from build123d import *

# Parameters (mm, degrees)
BOSS_EXTRUDE1_DEPTH = 20
FILLET1_R           = 5
FILLET2_R           = 2
FILLET3_R           = 1.5
SKETCH4_R           = 2.9
CUT_EXTRUDE3_DEPTH  = 2
SKETCH5_R           = 1.625
CUT_EXTRUDE4_DEPTH  = 89.064050596
CUT_EXTRUDE5_DEPTH  = 2.3


with BuildPart() as part:
    # Sketch1 → Boss-Extrude1 (new body)
    with BuildSketch(Plane(origin=(0, 0, 0), x_dir=(1, 0, 0), z_dir=(0, 1, 0))):
        with BuildLine():
            Line((2.5, 62.713850172), (5.5, 62.713850172))
            Line((5.5, 62.713850172), (5.5, 52.713850172))
            ThreePointArc((5.5, 52.713850172), (0, -53), (-5.5, 52.713850172))
            Line((-5.5, 52.713850172), (-5.5, 62.713850172))
            Line((-5.5, 62.713850172), (-2.5, 62.713850172))
            Line((-2.5, 62.713850172), (-2.5, 49.937460889))
            ThreePointArc((-2.5, 49.937460889), (0, -50), (2.5, 49.937460889))
            Line((2.5, 49.937460889), (2.5, 62.713850172))
        make_face()
    extrude(amount=BOSS_EXTRUDE1_DEPTH)

    # Fillet1
    fillet1_edges = [part.edges().sort_by_distance(p)[0] for p in [
        (-2.5, 10, -49.937460889),
        (2.5, 10, -49.937460889),
    ]]
    fillet(fillet1_edges, radius=FILLET1_R)

    # Fillet2
    fillet2_edges = [part.edges().sort_by_distance(p)[0] for p in [
        (5.5, 10, -52.713850172),
        (-5.5, 10, -52.713850172),
    ]]
    fillet(fillet2_edges, radius=FILLET2_R)

    # Fillet3
    fillet3_edges = [part.edges().sort_by_distance(p)[0] for p in [
        (2.5, 0, -58.600043483),
        (0, 0, 50),
        (0, 20, 50),
        (-2.5, 0, -58.600043483),
        (-3.731108193, 0, -51.200593091),
        (3.731108193, 0, -51.200593091),
        (-2.5, 20, -58.600043483),
        (-3.731108193, 20, -51.200593091),
        (3.731108193, 20, -51.200593091),
        (2.5, 20, -58.600043483),
    ]]
    fillet(fillet3_edges, radius=FILLET3_R)

    # Sketch4 → Cut-Extrude3 (cut)
    with BuildSketch(Plane.ZY.offset(5.5)):
        with Locations((-58.600043483, 15)):
            Circle(SKETCH4_R)
        with Locations((-58.600043483, 5)):
            Circle(SKETCH4_R)
    extrude(amount=-CUT_EXTRUDE3_DEPTH, mode=Mode.SUBTRACT)

    # Sketch5 → Cut-Extrude4 (cut, through all)
    with BuildSketch(Plane.ZY.offset(5.5)):
        with Locations((-58.600043483, 15)):
            Circle(SKETCH5_R)
        with Locations((-58.600043483, 5)):
            Circle(SKETCH5_R)
    extrude(amount=-CUT_EXTRUDE4_DEPTH, mode=Mode.SUBTRACT)

    # Sketch6 → Cut-Extrude5 (cut)
    with BuildSketch(Plane.ZY.offset(5.5)):
        Polygon((-55.338014462, 15), (-56.969028973, 17.825), (-60.231057994, 17.825), (-61.862072504, 15), (-60.231057994, 12.175), (-56.969028973, 12.175), align=None)
        Polygon((-55.338014462, 5), (-56.969028973, 7.825), (-60.231057994, 7.825), (-61.862072504, 5), (-60.231057994, 2.175), (-56.969028973, 2.175), align=None)
    extrude(amount=-CUT_EXTRUDE5_DEPTH, mode=Mode.SUBTRACT)


solid = part.part
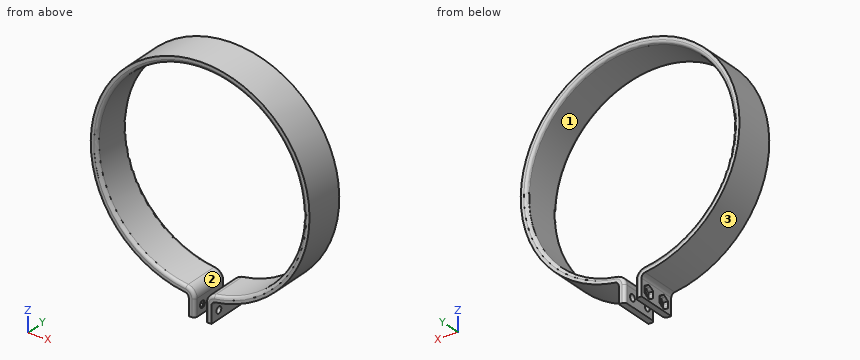
Geometry: final body of the model. Coordinates: model frame, mm. Face numbers are marked on the shaded views. Give positions to 0.01 mm unless a question says otherwise; leave off trailing zeros. Write each loop counter-clockwise with the first axis right and the second up, starting at its lowest first coordinate (ties: lowest second). Pieces come first, ordered by that corner, then holes. Notation, with made-up numbers: M 81.25,63 L 115.25,63 A14 ccw 115.25,79 Z; hole C 74.25,-15.75 d1. An arc over 180 degrees is marked long. Answer in a Markdown table with one row per item. Add a question column.
(1) Section A-A on y = 10.5. Return loops of the section in (x, z), and give its area (3 significant figures).
(2) First-contact query: pin 1 (2.5 mm diameter, centred on y = 10, z = -57.5, fed in from -X); pin 2 (2 mm diameter, centred on x = 11, y = 5.5, fed in from +Z); pin 3 (8 mm diameter, centred on y = 10, z = 29.5, fed in from -X); pin 4 (10 mm diameter, centred on x = -38.5, z = -22.5, fed in from +Y). Flat tips, straight axial feed; report the tip coordinate or a pass-through.
(3) Mould query, pull axis X, two halves, no side actions, for the marked faces 1, 2 and 3. Classes: +X half, -X half, draft (parallel to the pull), parting line (faces both ways), or undercut.
(4) Ray query, line 1 (X direction, y = 1.25, z = -0.5); line 2 (Z direction, x = 0, y = 9); line 3 (X direction, y = 11.25, z = 17). Return the intervals inside material, ascending.
(5) Section B-B on x = 0. Return loops of the section in (y, z), and give its area (3 significant figures).
Result set:
| question | item | result |
|---|---|---|
| 1 | outline | M -7.23,-52.5 A2 cw -5.5,-54.49 L -5.5,-62.71 L -2.5,-62.71 L -2.5,-54.49 A5 ccw -6.82,-49.53 A50 cw long 6.82,-49.53 A5 ccw 2.5,-54.49 L 2.5,-62.71 L 5.5,-62.71 L 5.5,-54.49 A2 cw 7.23,-52.5 A53 ccw long Z |
| 1 | area | 1,010 mm^2 |
| 2 | pin 1 | stops at x = -5.5 |
| 2 | pin 2 | stops at z = 52.05 |
| 2 | pin 3 | stops at x = -46.46 |
| 2 | pin 4 | passes through |
| 3 | face 1 | undercut |
| 3 | face 2 | undercut |
| 3 | face 3 | parting line |
| 4 | line 1 | x = -53 to -50.02, 50.02 to 53 |
| 4 | line 2 | z = 50 to 53 |
| 4 | line 3 | x = -50.2 to -47.02, 47.02 to 50.2 |
| 5 | outline | M 0,51.5 A1.5 ccw 1.5,50 L 18.5,50 A1.5 ccw 20,51.5 L 20,53 L 0,53 Z |
| 5 | area | 59.0 mm^2 |
